```python
from build123d import *

# Parameters (mm, degrees)
PAD007_DEPTH    = 5.6
SKETCH011_R     = 1.6
POCKET002_DEPTH = 2
SKETCH012_R     = 1.6
POCKET003_DEPTH = 2
FILLET001_R     = 1.2


with BuildPart() as part:
    # Sketch010 → Pad007 (new body)
    with BuildSketch(Plane.XZ):
        with BuildLine():
            Line((0, 4.120568), (0, 14))
            Line((2, 14), (0, 14))
            Line((2, 14), (2, 3.564131))
            ThreePointArc((2, 3.564131), (2.468629, 2.43276), (3.6, 1.964131))
            Line((3.6, 1.964131), (10.5, 1.964131))
            Line((10.5, 1.964131), (10.5, 0))
            Line((10.5, 0), (4.333415, 0))
            Line((4.333415, 0), (4.333415, 0.4))
            ThreePointArc((0.4, 4.120568), (1.368035, 1.204479), (4.333415, 0.4))
            Line((0, 4.120568), (0.4, 4.120568))
        make_face()
    extrude(amount=PAD007_DEPTH)

    # Sketch011 (on Face4 of Pad007) → Pocket002 (cut)
    with BuildSketch(Plane(origin=(2, 0, 0), x_dir=(0, 0, 1), z_dir=(1, 0, 0))):
        with Locations((10.7, 2.8)):
            Circle(SKETCH011_R)
    extrude(amount=-POCKET002_DEPTH, mode=Mode.SUBTRACT)

    # Sketch012 (on Face11 of Pocket002) → Pocket003 (cut)
    with BuildSketch(Plane(origin=(0, 0, 1.964131), x_dir=(-1, 0, 0), z_dir=(0, 0, 1))):
        with Locations((-7.5, 2.8)):
            Circle(SKETCH012_R)
    extrude(amount=-POCKET003_DEPTH, mode=Mode.SUBTRACT)

    # Fillet001
    fillet001_edges = [part.edges().sort_by_distance(p)[0] for p in [
        (1, 0, 14),
        (1, -5.6, 14),
        (10.5, -5.6, 0.982065),
        (10.5, 0, 0.982065),
    ]]
    fillet(fillet001_edges, radius=FILLET001_R)


with BuildPart() as part_1:
    # Body005 placement: moved
    add(part.part.moved(Location((1.6, 28.6, 0))))


solid = part_1.part
```
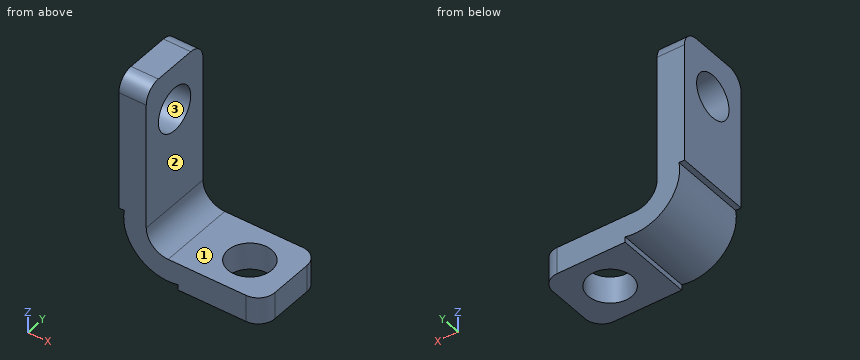
CAD build for the part. Positions are in the model's coordinates, mm. Face numbers are marked on the shaded views. Coordinates: 2 decimals unless noted, no trailing zeros. Loops run counter-clockwise (first coordinate to the right, second up) from the corner with the lowest first, then second, coordinate; pieces in that order, holes last. Notation, with made-up numbers: (67, 74.25) - (76, 74.25) arc R14 cw to (76, 88.25) - close; hole circle Ø3 at (-34.5, 53). An arc over 180 degrees is marked (long way). Return JSON: item names as keys, results as strings.
1. Mould opens along Z. For the marked faces 1, 2 and 3 say: released by +Z, released by -Z, zero draft, split by the parting line, or undercut.
Result:
{"face 1": "released by +Z", "face 2": "zero draft", "face 3": "undercut"}
2. Band-saw the part on B-B (z = 10.7). Give the cut face in (x, y), and give its area (3 significant figures).
Result:
{"outline": "(1.6, 23) - (3.6, 23) - (3.6, 24.2) - (1.6, 24.2) - close; (1.6, 27.4) - (3.6, 27.4) - (3.6, 28.6) - (1.6, 28.6) - close", "area": "4.80 mm2"}
3. Band-saw the part on A-A (y = 25.8). Give the cut face in (x, z).
Result:
{"outline": "(1.6, 4.12) - (2, 4.12) arc R3.25 ccw to (5.93, 0.4) - (5.93, 0) - (7.5, 0) - (7.5, 1.96) - (5.2, 1.96) arc R1.6 cw to (3.6, 3.56) - (3.6, 9.1) - (1.6, 9.1) - close; (1.6, 12.3) - (3.6, 12.3) - (3.6, 14) - (1.6, 14) - close; (10.7, 0) - (12.1, 0) - (12.1, 1.96) - (10.7, 1.96) - close"}
4. Band-saw the part on C-C (x = 9.1). Give the cut face in (y, z).
Result:
{"outline": "(23, 0) - (24.2, 0) - (24.2, 1.96) - (23, 1.96) - close; (27.4, 0) - (28.6, 0) - (28.6, 1.96) - (27.4, 1.96) - close"}
5. Drop flat-ended pins along their axis: pin 1 (3 mm diameter, centred on y = 25.8, z = 10.7, fed in from +X); pin 2 (1.7 mm diameter, centred on x = 7.5, y = 25, fed in from +Z). Give the stop position or say it passes through.
Result:
{"pin 1": "passes through", "pin 2": "stops at z = 1.96"}
6. Band-saw the part on D-D (x = 3). Give the cut face in (y, z).
Result:
{"outline": "(23, 1.17) - (28.6, 1.17) - (28.6, 12.8) arc R1.2 ccw to (27.4, 14) - (24.2, 14) arc R1.2 ccw to (23, 12.8) - close; hole circle Ø3.2 at (25.8, 10.7)"}
7. Probe L1, parallel to Y at x = 2.8, z = 10.7; L2, parallel to X at y = 26, z = 5.5; L3, parallel to Z at x = 6.5, y = 23.5. List the from-to ranges inside material, lowest first. Write a range as from..to.
Result:
{"L1": "y = 23..24.2, 27.4..28.6", "L2": "x = 1.6..3.6", "L3": "z = 0..1.96"}
